Read the model definition and answer for the solid it produces. Units are mm, in the model's axes. A direction names the side the tool comes from. Round coordinates to 2 decimals unless told otherwise and drop trailing zeros. Loops run counter-clockwise (first coordinate to the right, second up) from the corner with the lowest first, then second, coordinate; pieces in that order, holes last. Notation, with made-up numbers: M 49.25,-9.5 L 68.25,-9.5 A23 ccw 68.25,21.5 Z; hole C 49.25,-14.5 d1. An arc over 180 degrees is marked long. Answer as CSV lines item,"result".
Autodesk Inventor part; units mm, degrees
ref_plane "YZ Plane" through (0, 0, 0) normal (1, 0, 0) x (0, 1, 0)
ref_plane "XZ Plane" through (0, 0, 0) normal (0, 1, 0) x (-1, 0, 0)
ref_plane "XY Plane" through (0, 0, 0) normal (0, 0, 1) x (1, 0, 0)
sketch "Sketch1" plane through (0, 0, 0) normal (0, 0, 1) x (1, 0, 0)
  line L0 (0, 0) -> (220, 0) construction
  line L1 (220, 0) -> (220, 9) construction
  line L2 (220, 9) -> (0, 9) construction
  line L3 (0, 9) -> (0, 0) construction
  line L4 (0, 9) -> (90.94, 295.0593) construction
  line L5 (129.06, 295.0593) -> (220, 9) construction
  circle A0 centre (110, 289) radius 11 construction
  line L6 (96.1101, 281.616) -> (103.5522, 305.0259) construction
  arc A1 (129.06, 295.0593) -> (90.94, 295.0593) centre (110, 289) ccw construction
  line L7 (99, 275.5567) -> (99, 269.1274) construction
  line L8 (110, 289) -> (110, 143) construction
  line L9 (130, 289) -> (130, 143)
  line L10 (90, 143) -> (90, 289)
  arc A2 (130, 289) -> (90, 289) centre (110, 289) ccw
  arc A3 (90, 143) -> (130, 143) centre (110, 143) ccw
  line L11 (292.2692, 143) -> (292.2692, 247) construction
  line L12 (312.2692, 143) -> (312.2692, 247) construction
  line L13 (272.2692, 247) -> (272.2692, 143) construction
  arc A4 (272.2692, 143) -> (312.2692, 143) centre (292.2692, 143) ccw construction
  arc A5 (312.2692, 247) -> (272.2692, 247) centre (292.2692, 247) ccw construction
  arc A6 (90, 289) -> (130, 289) centre (110, 289) ccw construction
  line L14 (101.1908, 269) -> (118.8092, 269) construction
  line L15 (211.2941, 267) -> (373.2442, 267) construction
  line L16 (211.2941, 143) -> (373.2442, 143) construction
  line L17 (292.2692, 143) -> (292.2692, 39) construction
  line L18 (312.2692, 143) -> (312.2692, 39) construction
  line L19 (272.2692, 39) -> (272.2692, 143) construction
  arc A7 (312.2692, 143) -> (272.2692, 143) centre (292.2692, 143) ccw construction
  arc A8 (272.2692, 39) -> (312.2692, 39) centre (292.2692, 39) ccw construction
  line L20 (211.2941, 19) -> (373.2442, 19) construction
  circle A9 centre (110, 289) radius 11
  circle A10 centre (110, 143) radius 11
  point P0 (110, 0)
  point P1 (110, 216)
  point P2 (110, 309)
  point P3 (292.2692, 195)
  point P4 (110, 269)
  point P5 (110, 269)
  point P6 (292.2692, 267)
  dimension "d0" = 9
  dimension "d1" = 220
  dimension "d2" = 22
  dimension "d3" = 280
  dimension "d4" = 9
  dimension "d7" = 40
  dimension "d8" = 40
  dimension "pendgap" = 2
  dimension "abovethefloor" = 10
  dimension "d11" = 104
  dimension "d12" = 146
  dimension "d14" = 22
extrude "Extrusion2" add sketch "Sketch1" along normal blind 7
sketch "Sketch3" plane through (0, 0, 7) normal (0, 0, 1) x (1, 0, 0)
  line L0 (110, 175) -> (110, 257) construction
  line L1 (90, 289) -> (90, 143)
  line L2 (121, 175) -> (121, 257)
  line L3 (99, 257) -> (99, 175)
  arc A0 (99, 175) -> (121, 175) centre (110, 175) ccw
  arc A1 (121, 257) -> (99, 257) centre (110, 257) ccw
  line L4 (110, 268) -> (110, 278) construction
  circle A2 centre (110, 289) radius 11
  circle A3 centre (110, 289) radius 11 construction
  circle A4 centre (110, 143) radius 11
  point P0 (0, 0)
  point P1 (110, 216)
  point P2 (90, 216)
  dimension "d18" = 10
extrude "Extrusion3" cut sketch "Sketch3" against normal blind 6
properties part number "DBP-2-pendulum1"
1) Find section D-D, the plane y = 207.5. Give the vertices of the cut face in (x, z), then the cut area to 3 significant figures.
Evaluation:
outline,"M 90,0 L 130,0 L 130,7 L 121,7 L 121,1 L 99,1 L 99,7 L 90,7 Z"
area,"148 mm^2"
2) Each of these flat-tipped pins is pushed along its axis until it touches: P1, Ø3, axis at x = 101, z = 6, coming from the +Y side; P2, Ø20, axis at x = 110, y = 143, coming from the -Z side; P3, Ø5, axis at x = 110.5, y = 250, coming from the +Z side. Where does it stop, or does it pass through?
Evaluation:
P1,"stops at y = 307.54"
P2,"passes through"
P3,"stops at z = 1"
3) Find section C-C, the plane y = 292. Give the vertices of the cut face in (x, z), then the cut area to 3 significant figures.
Evaluation:
outline,"M 90.23,0 L 99.42,0 L 99.42,7 L 90.23,7 Z; M 120.58,0 L 129.77,0 L 129.77,7 L 120.58,7 Z"
area,"129 mm^2"
4) Determine the mould class of faces 1 (the flat face through (99, 217, 4)), 2 (the flat face through (110, 217, 0)), 3 (the cylindrical face through (101.89, 135.57, 3.45)), 4 (the flat face through (130, 217, 3)) for opening direction X: released by +X, released by -X, zero draft, split by the parting line, or undercut.
Evaluation:
face 1,"undercut"
face 2,"zero draft"
face 3,"undercut"
face 4,"released by +X"
5) Straight lines are drawn through the part: line 1 (Y direction, x = 110, z = 2.75); line 2 (X direction, y = 219, z = 2.5); line 3 (Z direction, x = 102, y = 204.5). For each, find the intervals that lie inside material, in ascending order.
Evaluation:
line 1,"y = 123 to 132, 154 to 164, 268 to 278, 300 to 309"
line 2,"x = 90 to 99, 121 to 130"
line 3,"z = 0 to 1"
6) Find section B-B, the plane z = 5. Give the vertices of the cut face in (x, y).
Evaluation:
outline,"M 90,143 A20 ccw 130,143 L 130,289 A20 ccw 90,289 Z; hole C 110,143 d22; hole M 99,175 A11 ccw 121,175 L 121,257 A11 ccw 99,257 Z; hole C 110,289 d22"
7) Find section A-A, the plane x = 106. Give the vertices of the cut face in (y, z), then the cut area to 3 significant figures.
Evaluation:
outline,"M 123.4,0 L 132.75,0 L 132.75,7 L 123.4,7 Z; M 153.25,0 L 278.75,0 L 278.75,7 L 267.25,7 L 267.25,1 L 164.75,1 L 164.75,7 L 153.25,7 Z; M 299.25,0 L 308.6,0 L 308.6,7 L 299.25,7 Z"
area,"394 mm^2"
8) A tool of negligible diameter and unlimited length cuts with its end or side. For faces 5 (the cylindrical face through (110, 268, 4)), 6 (the cylindrical face through (110, 309, 3)), from which of +Z, -Z, +X, -X, +Y, -Y can it reach the whole face along a straight path? Write none if from no direction.
Evaluation:
face 5,"+Z"
face 6,"+Z, -Z, +Y"
